Design review of the part built by this model. Coordinates are the model's own, in mm. A direction names the side the tool comes from. Give positions to 0.01 mm unless a question says otherwise; leave off trailing zeros. Use CSV: the item, a comma, the result in double quotes. Start each with the question number.
Item 1: For faces 1 (the face through (-72, -3.915, 1)), 2 (the face through (26, -3.915, 1)), 3 (the face through (-23, -3.915, 1)), 4 (the face through (42.263, 11, 1)), list the 3-axis set-ups (+Z, -Z, +X, -X, +Y, -Y) from which the entire face can be reached by the end or side of a thin tool; tool diameter is ignored.
Item 2: The part is to be moulded in two halves that separate along X. For faces 5 (the face through (26, 2.085, 1)), 6 (the face through (-56, -2.115, 1)), 7 (the face through (-88.237, -5, 1)), say which applies: +X half, -X half, draft (parallel to the pull), parting line (faces both ways), or undercut.
Item 3: Wall thickness on line 1 along X through (y, z) = (0.5, 2.2); line 2 along X through (y, z) = (7.5, 0.25): over which ranges is each line inside the solid? List them lowest first. Write a range as from..to.
Item 4: We need section A-A (x = -41). Count the separate pieces of the cut face and the enclosed holes in it, plus the area to 3 significant figures.
from build123d import *

# Parameters (mm, degrees)
F0_W     = 63
F0_H     = 0.4
F1_DEPTH = 3


with BuildPart() as f1:
    # F0 (on Top) → F1 (new body)
    with BuildSketch(Plane.XY):
        Polygon((42.2626923621, 7.6849870265), (42.2626923621, 14.0849870265), (-88.2373076379, 14.0849870265), (-88.2373076379, 7.6849870265), (-55.9873076379, 7.6849870265), (-55.9873076379, 7.2849870265), (-88.2373076379, 7.2849870265), (-88.2373076379, 4.8849870265), (-55.9873076379, 4.8849870265), (-55.9873076379, 4.4849870265), (-88.2373076379, 4.4849870265), (-88.2373076379, 2.0849870265), (-55.9873076379, 2.0849870265), (-55.9873076379, 1.6849870265), (-88.2373076379, 1.6849870265), (-88.2373076379, -0.7150129735), (-55.9873076379, -0.7150129735), (-55.9873076379, -1.1150129735), (-88.2373076379, -1.1150129735), (-88.2373076379, -3.5150129735), (-55.9873076379, -3.5150129735), (-55.9873076379, -3.9150129735), (-88.2373076379, -3.9150129735), (-88.2373076379, -6.3150129735), (-55.9873076379, -6.3150129735), (-55.9873076379, -6.7150129735), (-88.2373076379, -6.7150129735), (-88.2373076379, -11.7150129735), (42.2626923621, -11.7150129735), (42.2626923621, -6.7150129735), (10.0126923621, -6.7150129735), (10.0126923621, -6.3150129735), (42.2626923621, -6.3150129735), (42.2626923621, -3.9150129735), (10.0126923621, -3.9150129735), (10.0126923621, -3.5150129735), (42.2626923621, -3.5150129735), (42.2626923621, -1.1150129735), (10.0126923621, -1.1150129735), (10.0126923621, -0.7150129735), (42.2626923621, -0.7150129735), (42.2626923621, 1.6849870265), (10.0126923621, 1.6849870265), (10.0126923621, 2.0849870265), (42.2626923621, 2.0849870265), (42.2626923621, 4.4849870265), (10.0126923621, 4.4849870265), (10.0126923621, 4.8849870265), (42.2626923621, 4.8849870265), (42.2626923621, 7.2849870265), (10.0126923621, 7.2849870265), (10.0126923621, 7.6849870265), align=None)
        with Locations((-55.2373076379, -5.1150129735)):
            Rectangle(F0_W, F0_H, mode=Mode.SUBTRACT)
        with Locations((-55.2373076379, -2.3150129735)):
            Rectangle(F0_W, F0_H, mode=Mode.SUBTRACT)
        with Locations((-55.2373076379, 0.4849870265)):
            Rectangle(F0_W, F0_H, mode=Mode.SUBTRACT)
        with Locations((-22.9873076379, -6.5150129735)):
            Rectangle(F0_W, F0_H, mode=Mode.SUBTRACT)
        with Locations((-22.9873076379, -3.7150129735)):
            Rectangle(F0_W, F0_H, mode=Mode.SUBTRACT)
        with Locations((9.2626923621, -5.1150129735)):
            Rectangle(F0_W, F0_H, mode=Mode.SUBTRACT)
        with Locations((9.2626923621, -2.3150129735)):
            Rectangle(F0_W, F0_H, mode=Mode.SUBTRACT)
        with Locations((-22.9873076379, -0.9150129735)):
            Rectangle(F0_W, F0_H, mode=Mode.SUBTRACT)
        with Locations((9.2626923621, 0.4849870265)):
            Rectangle(F0_W, F0_H, mode=Mode.SUBTRACT)
        with Locations((-55.2373076379, 3.2849870265)):
            Rectangle(F0_W, F0_H, mode=Mode.SUBTRACT)
        with Locations((-55.2373076379, 6.0849870265)):
            Rectangle(F0_W, F0_H, mode=Mode.SUBTRACT)
        with Locations((-55.2373076379, 8.8849870265)):
            Rectangle(F0_W, F0_H, mode=Mode.SUBTRACT)
        with Locations((-22.9873076379, 1.8849870265)):
            Rectangle(F0_W, F0_H, mode=Mode.SUBTRACT)
        with Locations((9.2626923621, 3.2849870265)):
            Rectangle(F0_W, F0_H, mode=Mode.SUBTRACT)
        with Locations((-22.9873076379, 4.6849870265)):
            Rectangle(F0_W, F0_H, mode=Mode.SUBTRACT)
        with Locations((-22.9873076379, 7.4849870265)):
            Rectangle(F0_W, F0_H, mode=Mode.SUBTRACT)
        with Locations((9.2626923621, 6.0849870265)):
            Rectangle(F0_W, F0_H, mode=Mode.SUBTRACT)
        with Locations((9.2626923621, 8.8849870265)):
            Rectangle(F0_W, F0_H, mode=Mode.SUBTRACT)
    extrude(amount=F1_DEPTH)


solid = f1.part
Results found:
1,face 1,"+Z, -Z, -X"
1,face 2,"+Z, -Z, +X"
1,face 3,"+Z, -Z"
1,face 4,"+Z, -Z, +X, +Y, -Y"
2,face 5,"draft"
2,face 6,"undercut"
2,face 7,"-X half"
3,line 1,"-88.24..-86.74, -23.74..-22.24, 40.76..42.26"
3,line 2,"-55.99..-54.49, 8.51..10.01"
4,separate pieces,"13"
4,enclosed holes,"0"
4,area,"63.0 mm²"
